Verification items for the finished model (mm, model axes). Give positions to 0.01 mm unless a question says otherwise; leave off trailing zeros. Write each loop counter-clockwise with the first axis right and the second up, starting at its lowest first coordinate (ties: lowest second). Pieces come first, ordered by that corner, then holes. Notation, with made-up numbers: (63.5, 70) - (102.5, 70) arc R25 ccw to (102.5, 91) - close; hole circle Ø5 at (25.5, -37). An arc over 180 degrees is marked (long way). Put each result on its own line as item: value.
from build123d import *

# Parameters (mm, degrees)
SKETCH1_W           = 290
SKETCH1_H           = 154.65
BOSS_EXTRUDE1_DEPTH = 3
CUT_EXTRUDE1_DEPTH  = 165.356793669
SKETCH3_W           = 10
SKETCH3_H           = 15
CUT_EXTRUDE2_DEPTH  = 3
SKETCH5_W           = 40
SKETCH5_H           = 9
CUT_EXTRUDE3_DEPTH  = 3
SKETCH6_W           = 20
SKETCH6_H           = 30
CUT_EXTRUDE4_DEPTH  = 3


with BuildPart() as part:
    # Sketch1 → Boss-Extrude1 (new body)
    with BuildSketch(Plane(origin=(0, 0, 0), x_dir=(1, 0, 0), z_dir=(0, 1, 0))):
        Rectangle(SKETCH1_W, SKETCH1_H)
    extrude(amount=BOSS_EXTRUDE1_DEPTH)

    # Sketch2 → Cut-Extrude1 (cut, through all)
    with BuildSketch(Plane(origin=(0, 3, 0), x_dir=(1, 0, 0), z_dir=(0, 1, 0))):
        Polygon((53, 77.325), (-16, 77.325), (-16, 71.325), (-10.5, 71.325), (-10.5, 36.825), (10.5, 36.825), (10.5, 35.325), (19.5, 35.325), (39.5, 35.325), (53, 35.325), align=None)
    extrude(amount=-CUT_EXTRUDE1_DEPTH, mode=Mode.SUBTRACT)

    # Sketch3 → Cut-Extrude2 (cut)
    with BuildSketch(Plane(origin=(0, 3, 0), x_dir=(1, 0, 0), z_dir=(0, 1, 0))):
        with Locations((58, 63.825)):
            Rectangle(SKETCH3_W, SKETCH3_H)
        with Locations((58, 48.825)):
            Rectangle(SKETCH3_W, SKETCH3_H)
    extrude(amount=-CUT_EXTRUDE2_DEPTH, mode=Mode.SUBTRACT)

    # Sketch5 → Cut-Extrude3 (cut)
    with BuildSketch(Plane(origin=(0, 0, 0), x_dir=(-1, 0, 0), z_dir=(0, -1, 0))):
        with Locations((-125, -72.825)):
            Rectangle(SKETCH5_W, SKETCH5_H)
    extrude(amount=-CUT_EXTRUDE3_DEPTH, mode=Mode.SUBTRACT)

    # Sketch6 → Cut-Extrude4 (cut)
    with BuildSketch(Plane(origin=(0, 3, 0), x_dir=(1, 0, 0), z_dir=(0, 1, 0))):
        with Locations((135, -53.325)):
            Rectangle(SKETCH6_W, SKETCH6_H)
    extrude(amount=-CUT_EXTRUDE4_DEPTH, mode=Mode.SUBTRACT)


solid = part.part
Q1. Section check D-D, the plane x = 115.5. Record the cut outline in (y, z) (3 decimals), plus the area to 3 significant figures.
Answers follow:
outline: (0, -77.325) - (3, -77.325) - (3, 68.325) - (0, 68.325) - close
area: 437 mm2
Q2. Section check C-C, the plane z = 41. Record the cut outline in (x, y).
Answers follow:
outline: (-145, 0) - (125, 0) - (125, 3) - (-145, 3) - close
Q3. Scan lines: line 1 along X through (y, z) = (2.8, -53.5); line 2 along X through (y, z) = (2.4, -37.5); line 3 along X through (y, z) = (0.2, 48). Record each from-to range of solid material in increasing order.
Answers follow:
line 1: x = -145 to -10.5, 63 to 145
line 2: x = -145 to -10.5, 53 to 145
line 3: x = -145 to 125
Q4. Section check A-A, the plane z = -59.5. Record the cut outline in (x, y), plus the area to 4 significant figures.
Answers follow:
outline: (-145, 0) - (-10.5, 0) - (-10.5, 3) - (-145, 3) - close; (63, 0) - (145, 0) - (145, 3) - (63, 3) - close
area: 649.5 mm2
Q5. Section check B-B, the plane y = 1.6. Record the cut outline in (x, z) (3 decimals).
Answers follow:
outline: (-145, -77.325) - (-16, -77.325) - (-16, -71.325) - (-10.5, -71.325) - (-10.5, -36.825) - (10.5, -36.825) - (10.5, -35.325) - (53, -35.325) - (53, -41.325) - (63, -41.325) - (63, -71.325) - (53, -71.325) - (53, -77.325) - (145, -77.325) - (145, 38.325) - (125, 38.325) - (125, 68.325) - (105, 68.325) - (105, 77.325) - (-145, 77.325) - close
Q6. Go/stop test with flat-tipped pins: pin 1 Ø1.5 at (x, y) = (110.5, 1.5) entering from +Z (3 decimals); pin 2 Ø1.5 at (x, y) = (135.5, 1) entering from +Z (3 decimals); pin 3 Ø1 at (x, y) = (18.5, 1.5) entering from -Z (3 decimals). Record where each tip stops, or that it passes through.
Answers follow:
pin 1: stops at z = 68.325
pin 2: stops at z = 38.325
pin 3: stops at z = -35.325
